```python
from build123d import *

# Parameters (mm, degrees)
SKETCH2_W           = 76.2
SKETCH2_H           = 76.2
BOSS_EXTRUDE2_DEPTH = 2.54
SKETCH5_R           = 2.286
CUT_EXTRUDE1_DEPTH  = 2.54
SKETCH6_R           = 3.175
CUT_EXTRUDE2_DEPTH  = 2.54
FILLET3_R           = 2.54


with BuildPart() as part:
    # Sketch2 → Boss-Extrude2 (new body)
    with BuildSketch(Plane(origin=(0, 0, 0), x_dir=(1, 0, 0), z_dir=(0, 1, 0))):
        Rectangle(SKETCH2_W, SKETCH2_H)
    extrude(amount=BOSS_EXTRUDE2_DEPTH)

    # Sketch5 → Cut-Extrude1 (cut)
    with BuildSketch(Plane(origin=(0, 2.54, 0), x_dir=(1, 0, 0), z_dir=(0, 1, 0))):
        with Locations((-32.512, 32.512)):
            Circle(SKETCH5_R)
        with Locations((32.512, 32.512)):
            Circle(SKETCH5_R)
        with Locations((32.512, -32.512)):
            Circle(SKETCH5_R)
        with Locations((-32.512, -32.512)):
            Circle(SKETCH5_R)
    extrude(amount=-CUT_EXTRUDE1_DEPTH, mode=Mode.SUBTRACT)

    # Sketch6 → Cut-Extrude2 (cut)
    with BuildSketch(Plane(origin=(0, 2.54, 0), x_dir=(1, 0, 0), z_dir=(0, 1, 0))):
        Circle(SKETCH6_R)
    extrude(amount=-CUT_EXTRUDE2_DEPTH, mode=Mode.SUBTRACT)

    # Fillet3
    fillet3_edges = [part.edges().sort_by_distance(p)[0] for p in [
        (38.1, 1.27, 38.1),
        (-38.1, 1.27, 38.1),
        (-38.1, 1.27, -38.1),
        (38.1, 1.27, -38.1),
    ]]
    fillet(fillet3_edges, radius=FILLET3_R)


solid = part.part
```
Geometry: final body of the model. Coordinates: model frame, mm. Round coordinates to 2 decimals unless told otherwise and drop trailing zeros. Write each loop counter-clockwise with the first axis right and the second up, starting at its lowest first coordinate (ties: lowest second). Pieces come first, ordered by that corner, then holes.
Item 1: Section query D-D (x = 33). Return loops of the section in (y, z).
Item 2: Material intervals for L1, parallel to Z at x = -32.5, y = 0.95; L2, parallel to Z at x = 0, y = 0.85 (3 decimals), sorted ascending.
Item 3: Section query A-A (x = 0). Return loops of the section in (y, z) (3 decimals).
Item 4: Section query B-B (z = 0). Return loops of the section in (x, y) (3 decimals), plus the area to 3 significant figures.
Item 5: Mould query, pull axis Z, two halves, no side actions, for faces 1 (the face through (0, 1, -38.1)), 2 (the face through (-0.69, 1.29, 3.1)), 3 (the face through (-1, 0, -9)). Classes: +Z half, -Z half, draft (parallel to the pull), parting line (faces both ways), or undercut.
Item 6: Pin query (flat end, axial travel): P1, Ø3.5, axis at x = 32.512, z = -32.512, coming from the -Y side. Return the tip coordinate at first contact, or that it passes through.
Item 7: Section query C-C (y = 0.6). Return loops of the section in (x, z) (3 decimals).
Completed:
1. outline: (0, -38.1) - (2.54, -38.1) - (2.54, -34.75) - (0, -34.75) - close; (0, -30.28) - (2.54, -30.28) - (2.54, 30.28) - (0, 30.28) - close; (0, 34.75) - (2.54, 34.75) - (2.54, 38.1) - (0, 38.1) - close
2. L1: z = -38.1 to -34.8, -30.23 to 30.23, 34.8 to 38.1
2. L2: z = -38.1 to -3.175, 3.175 to 38.1
3. outline: (0, -38.1) - (2.54, -38.1) - (2.54, -3.175) - (0, -3.175) - close; (0, 3.175) - (2.54, 3.175) - (2.54, 38.1) - (0, 38.1) - close
4. outline: (-38.1, 0) - (-3.175, 0) - (-3.175, 2.54) - (-38.1, 2.54) - close; (3.175, 0) - (38.1, 0) - (38.1, 2.54) - (3.175, 2.54) - close
4. area: 177 mm2
5. face 1: -Z half
5. face 2: undercut
5. face 3: draft
6. P1: passes through
7. outline: (-38.1, -35.56) arc R2.54 ccw to (-35.56, -38.1) - (35.56, -38.1) arc R2.54 ccw to (38.1, -35.56) - (38.1, 35.56) arc R2.54 ccw to (35.56, 38.1) - (-35.56, 38.1) arc R2.54 ccw to (-38.1, 35.56) - close; hole circle Ø4.572 at (-32.512, -32.512); hole circle Ø4.572 at (-32.512, 32.512); hole circle Ø6.35 at (0, 0); hole circle Ø4.572 at (32.512, -32.512); hole circle Ø4.572 at (32.512, 32.512)
